Here's how the part is built. I have some questions about the finished solid (model axes, mm). A direction names the side the tool comes from. Round coordinates to 2 decimals unless told otherwise and drop trailing zeros. Loops run counter-clockwise (first coordinate to the right, second up) from the corner with the lowest first, then second, coordinate; pieces in that order, holes last. Notation, with made-up numbers: M -23.5,15 L 20.5,15 A17 cw 20.5,46 Z; hole C 14,36.5 d1. An arc over 180 degrees is marked long. Use a Markdown table: item, result.
Autodesk Inventor part; units mm, degrees
ref_plane "YZ Plane" through (0, 0, 0) normal (1, 0, 0) x (0, 1, 0)
ref_plane "XZ Plane" through (0, 0, 0) normal (0, 1, 0) x (-1, 0, 0)
ref_plane "XY Plane" through (0, 0, 0) normal (0, 0, 1) x (1, 0, 0)
sketch "Sketch1" plane through (0, 0, 0) normal (0, 0, 1) x (1, 0, 0)
  circle A0 centre (0, 0) radius 3
  line L0 (-1.9284, 2.2981) -> (4.0304, 7.2981)
  line L1 (5.9588, 8) -> (33, 8)
  line L2 (35, 6) -> (35, 4)
  line L3 (33, 2) -> (8.1426, 2)
  line L4 (6.2142, 1.2981) -> (1.9284, -2.2981)
  arc A1 (5.9588, 8) -> (4.0304, 7.2981) centre (5.9588, 5) ccw
  arc A2 (8.1426, 2) -> (6.2142, 1.2981) centre (8.1426, -1) ccw
  arc A3 (35, 6) -> (33, 8) centre (33, 6) ccw
  arc A4 (33, 2) -> (35, 4) centre (33, 4) ccw
  circle A5 centre (0, 0) radius 1.75
  point P0 (35, 8)
  point P1 (35, 2)
  dimension "d0" = 6
  dimension "d1" = 6
  dimension "d2" = 3
  dimension "d3" = 140
  dimension "d4" = 2
  dimension "d5" = 2
  dimension "d6" = 35
  dimension "d7" = 3.5
extrude "Extrusion1" add sketch "Sketch1" along normal blind 4
sketch "Sketch2" plane through (0, 0, 4) normal (0, 0, 1) x (1, 0, 0)
  line L0 (63, 2.75) -> (7, 2.75)
  line L1 (7, 2.75) -> (7, 7.25)
  line L2 (7, 7.25) -> (63, 7.25)
  line L3 (63, 7.25) -> (63, 2.75)
  line L4 (35, 4) -> (35, 6)
  line L5 (63, 2.75) -> (7, 7.25) construction
  line L6 (7, 2.75) -> (63, 7.25) construction
  point P0 (0, 0)
  point P1 (35, 5)
  dimension "d10" = 4.5
  dimension "d11" = 28
extrude "Extrusion2" cut sketch "Sketch2" against normal blind 1
properties part number "espcam-mount-2a"
Q1. We'd pull the mould along Y, two halves only. Please class faces 4 (the flat face through (19, 8, 2)), 5 (the flat face through (21, 2.75, 3.5)), 6 (the cylindrical face through (34.43, 2.6, 1.97)), 7 (the flat face through (16, 4, 0)): pulls with the +Y half, pulls with the -Y half, needs draft (parallel to the pull), parting line crosses it, or undercut.
Return value:
| item | result |
|---|---|
| face 4 | pulls with the +Y half |
| face 5 | undercut |
| face 6 | pulls with the -Y half |
| face 7 | needs draft |
Q2. Imagine slicing it at D-D, the plane y = 3.5. Please give me the cut outline in (x, z), then the cut area to 3 significant figures.
Return value:
| item | result |
|---|---|
| outline | M -0.5,0 L 34.94,0 L 34.94,3 L 7,3 L 7,4 L -0.5,4 Z |
| area | 114 mm^2 |
Q3. I need wall thicknesses on line 1 (Y direction, x = 23.5, z = 3.4); line 2 (Z direction, x = 19.5, y = 6); line 3 (X direction, y = 1, z = 2.05). Which ranges of each line are inside material? Lowest first, please. Write a range as from..to.
Return value:
| item | result |
|---|---|
| line 1 | y = 2..2.75, 7.25..8 |
| line 2 | z = 0..3 |
| line 3 | x = -2.83..-1.44, 1.44..5.86 |
Q4. Imagine slicing it at C-C, the plane x = 1. Please give me the cut outline in (y, z), then the cut area to 3 significant figures.
Return value:
| item | result |
|---|---|
| outline | M -2.83,0 L -1.44,0 L -1.44,4 L -2.83,4 Z; M 1.44,0 L 4.76,0 L 4.76,4 L 1.44,4 Z |
| area | 18.8 mm^2 |
Q5. Imagine slicing it at B-B, the plane y = -1. Please give me the cut outline in (x, z), then the cut area to 3 significant figures.
Return value:
| item | result |
|---|---|
| outline | M -2.83,0 L -1.44,0 L -1.44,4 L -2.83,4 Z; M 1.44,0 L 3.48,0 L 3.48,4 L 1.44,4 Z |
| area | 13.7 mm^2 |
Q6. Will these pins go through, and if not, where does the flat tip stop? P1, Ø2, axis at x = 20.5, z = 1, coming from the -Y side; P2, Ø1.4, axis at x = 26, y = 5, coming from the +Z side.
Return value:
| item | result |
|---|---|
| P1 | stops at y = 2 |
| P2 | stops at z = 3 |
Q7. Imagine slicing it at A-A, the plane z = 2.45. Please give me the cut outline in (x, y), then the cut area to 3 significant figures.
Return value:
| item | result |
|---|---|
| outline | M -1.93,2.3 A3 ccw 1.93,-2.3 L 6.21,1.3 A3 cw 8.14,2 L 33,2 A2 ccw 35,4 L 35,6 A2 ccw 33,8 L 5.96,8 A3 ccw 4.03,7.3 Z; hole C 0,0 d3.5 |
| area | 224 mm^2 |
Q8. For faces 1 (the flat face through (1.009, 4.763, 1.972)), 2 (the flat face through (21, 2, 2)), 3 (the flat face through (20.6, 7.25, 3.5)), which set-ups out of +Z, -Z, +X, -X, +Y, -Y let a thin tool reach every point of the face, with its end or its side?
Return value:
| item | result |
|---|---|
| face 1 | +Z, -Z, -X, +Y |
| face 2 | +Z, -Z, +X, -Y |
| face 3 | +Z, +X |
